Autodesk Inventor part; units mm, degrees
ref_plane "YZ Plane" through (0, 0, 0) normal (1, 0, 0) x (0, 1, 0)
ref_plane "XZ Plane" through (0, 0, 0) normal (0, 1, 0) x (-1, 0, 0)
ref_plane "XY Plane" through (0, 0, 0) normal (0, 0, 1) x (1, 0, 0)
sketch "Sketch1" plane through (0, 0, 0) normal (0, 1, 0) x (-1, 0, 0)
  circle A0 centre (0, 0) radius 6.15
  line L0 (10, 13) -> (-10, 13)
  line L1 (-10, 13) -> (-10, -13)
  line L2 (-10, -13) -> (10, -13)
  line L3 (10, -13) -> (10, 13)
  dimension "d0" = 12.3
  dimension "d1" = 10
  dimension "d2" = 10
  dimension "d3" = 13
  dimension "d4" = 13
extrude "Extrusion1" add sketch "Sketch1" along normal blind 15
sketch "Sketch2" plane through (10, 0, 13) normal (1, 0, 0) x (0, 0, -1)
  circle A0 centre (13, 6.5) radius 1.45
  line L0 (0, 0) -> (26, 0)
  line L1 (0, 0) -> (0, 15)
  point P0 (13, 0)
  dimension "d7" = 2.9
  dimension "d8" = 6.5
  dimension "d11" = 13
extrude "Extrusion2" cut sketch "Sketch2" against normal blind 55
sketch "Sketch3" plane through (10, 0, 13) normal (1, 0, 0) x (0, 0, -1)
  circle A0 centre (13, 6.5) radius 1.45
  line L0 (0, 0) -> (26, 0)
  line L1 (26, 0) -> (26, 15)
  line L2 (0, 15) -> (26, 15)
  line L3 (0, 0) -> (0, 15)
  circle A1 centre (13, 6.5) radius 5.45
  circle A2 centre (4, 6.5) radius 1.6
  circle A3 centre (22, 6.5) radius 1.6
  point P0 (13, 0)
  dimension "d16" = 4
  dimension "d21" = 3.2
  dimension "d22" = 3.2
  dimension "d23" = 4
  dimension "d24" = 4
extrude "Extrusion3" add sketch "Sketch3" along normal blind 15 contours A1
sketch "Sketch6" plane through (-10, 0, 13) normal (0, 0, 1) x (1, 0, 0)
  line L0 (0, 0) -> (0, 15)
  line L1 (0, 15) -> (5, 15)
  line L2 (5, 15) -> (5, 0)
  line L3 (5, 0) -> (0, 0)
  line L4 (0, 0) -> (0, 15)
  point P0 (10, 0)
  dimension "d31" = 5
extrude "Extrusion6" add sketch "Sketch6" along normal blind 5
sketch "Sketch7" plane through (10, 0, -13) normal (0, 0, -1) x (-1, 0, 0)
  line L0 (20, 0) -> (20, 15)
  line L1 (20, 15) -> (15, 15)
  line L2 (15, 15) -> (15, 0)
  line L3 (15, 0) -> (20, 0)
  line L4 (20, 0) -> (20, 15)
  point P0 (10, 0)
  dimension "d34" = 5
extrude "Extrusion7" add sketch "Sketch7" along normal blind 5
sketch "Sketch8" plane through (0, 0, 0) normal (0, -1, 0) x (1, 0, 0)
  line L0 (10, 13) -> (10, -13)
  line L1 (-10, 18) -> (-10, -18)
  line L2 (10, 13) -> (-10, 13)
  line L3 (-10, 13) -> (-10, 3)
  line L4 (-10, 3) -> (10, 3)
  line L5 (10, 3) -> (10, 13)
  line L6 (10, -13) -> (-5, -13)
  line L7 (10, -13) -> (-10, -13)
  line L8 (-10, -13) -> (-10, -3)
  line L9 (-10, -3) -> (10, -3)
  line L10 (10, -3) -> (10, -13)
  point P0 (0, 0)
  point P1 (10, -3)
  point P2 (-10, -3)
  dimension "d37" = 10
  dimension "d38" = 10
extrude "Extrusion8" add sketch "Sketch8" along normal blind 2 contours L0 L4 L1 L2 | L0 L6 L7 L1 L9
properties part number "Tube_innerhole_template_p1"
Geometry check sheet. Reference: the model listing, model coordinates, mm. A direction names the side the tool comes from. Coordinates: 2 decimals unless noted, no trailing zeros. Write each loop counter-clockwise with the first axis right and the second up, starting at its lowest first coordinate (ties: lowest second). Pieces come first, ordered by that corner, then holes. Notation, with made-up numbers: M 6,-27.75 L 36,-27.75 A27 ccw 36,11.25 Z; hole C 88.5,58.25 d1. An arc over 180 degrees is marked long. Answer as a JSON object with one key per item and string values.
1. Section check D-D, the plane y = 4. Enter the section's corners in (x, z).
Answers below:
{"outline": "M -10,-18 L -5,-18 L -5,-13 L 10,-13 L 10,-4.84 L 25,-4.84 L 25,4.84 L 10,4.84 L 10,13 L -5,13 L -5,18 L -10,18 Z; hole C 0,0 d12.3"}
2. Tool access check on faces 1 (the cylindrical face through (-5.68, 7.4, 2.36)), 2 (the flat face through (0, -1, 3)), 3 (the flat face through (-5, 8, -15)), 4 (the flat face through (-5, 8, 15)), 5 (the flat face through (-7, 0, 16)). Record the directions out of +Z, -Z, +X, -X, +Y, -Y that give a thin tool (end or side, any length) a straight path to the whole face; none if there is none.
Answers below:
{"face 1": "+Y", "face 2": "+X, -X, -Y", "face 3": "-Z, +X, +Y, -Y", "face 4": "+Z, +X, +Y, -Y", "face 5": "+Z, +X, -X, -Y"}
3. Section check A-A, the plane x = 0. Enter the section's corners in (y, z).
Answers below:
{"outline": "M -2,-13 L 15,-13 L 15,-6.15 L 0,-6.15 L 0,-3 L -2,-3 Z; M -2,3 L 0,3 L 0,6.15 L 15,6.15 L 15,13 L -2,13 Z"}
4. Go/stop test with flat-tipped pins: pin 1 Ø5 at (x, y) = (9.5, 5) entering from +Z; pin 2 Ø4 at (x, z) = (-7.5, -16) entering from -Y; pin 3 Ø4 at (y, z) = (6.5, 0) entering from -X; pin 4 Ø1.5 at (y, z) = (5.5, -15.5) entering from +X. Record where each tip stops, or that it passes through.
Answers below:
{"pin 1": "stops at z = 13", "pin 2": "stops at y = 0", "pin 3": "stops at x = -10", "pin 4": "stops at x = -5"}
5. Section check B-B, the plane z = 0. Enter the section's corners in (x, y), plus the area to 3 significant figures.
Answers below:
{"outline": "M -10,0 L -6.15,0 L -6.15,5.05 L -10,5.05 Z; M -10,7.95 L -6.15,7.95 L -6.15,15 L -10,15 Z; M 6.15,0 L 10,0 L 10,1.05 L 25,1.05 L 25,5.05 L 6.15,5.05 Z; M 6.15,7.95 L 25,7.95 L 25,11.95 L 10,11.95 L 10,15 L 6.15,15 Z", "area": "213 mm²"}
6. Section check C-C, the plane y = 6.5. Enter the section's corners in (x, z).
Answers below:
{"outline": "M -10,-18 L -5,-18 L -5,-13 L 10,-13 L 10,-5.45 L 25,-5.45 L 25,-1.45 L 5.98,-1.45 A6.15 cw -5.98,-1.45 L -10,-1.45 Z; M -10,1.45 L -5.98,1.45 A6.15 cw 5.98,1.45 L 25,1.45 L 25,5.45 L 10,5.45 L 10,13 L -5,13 L -5,18 L -10,18 Z"}
7. Draft check along Z on faces 6 (the flat face through (-7, 8, -18)), 7 (the flat face through (0, 0, 4)), 8 (the cylindrical face through (-7.96, 6.56, 1.45)), 9 (the cylindrical face through (17.395, 4.863, -5.198)). Enter one of: released by +Z, released by -Z, zero draft, split by the parting line, or undercut.
Answers below:
{"face 6": "released by -Z", "face 7": "undercut", "face 8": "undercut", "face 9": "split by the parting line"}
8. Scan lines: L1, parallel to Y at x = 7, z = 0; L2, parallel to Z at x = -7.8, y = 6.5; L3, parallel to Z at x = 0, y = 7. Record each from-to range of solid material in increasing order.
Answers below:
{"L1": "y = 0 to 5.05, 7.95 to 15", "L2": "z = -18 to -1.45, 1.45 to 18", "L3": "z = -13 to -6.15, 6.15 to 13"}
